For this review, take the finished solid that the model builds, in its own axes (mm). A direction names the side the tool comes from. Round coordinates to 2 decimals unless told otherwise and drop trailing zeros. Order: outer loops, then holes, each group sorted by start corner. A loop starts at its lowest first (then second) coordinate and runs counter-clockwise, first axis right, second up. Notation, with made-up numbers: M -36.75,42 L -19.75,42 A34 cw -19.75,72 Z; hole C -14,69.5 d3. An arc over 180 degrees is marked long. Put each result on its own line as item: value.
from build123d import *

# Parameters (mm, degrees)
BOSS_EXTRUDE1_DEPTH = 6.35


with BuildPart() as part:
    # Sketch1 → Boss-Extrude1 (new body)
    with BuildSketch(Plane(origin=(0, 0, 0), x_dir=(1, 0, 0), z_dir=(0, 1, 0))):
        with BuildLine():
            ThreePointArc((11.585828754, -34.373994235), (16.841756292, -62.617220967), (31.905828754, -87.078994235))
            Line((31.905828754, -87.078994235), (31.905828754, 39.921005765))
            Line((31.905828754, 39.921005765), (-120.494171246, 39.921005765))
            Line((-120.494171246, 39.921005765), (-120.494171246, -87.078994235))
            ThreePointArc((-120.494171246, -87.078994235), (-105.430098785, -62.617220967), (-100.174171246, -34.373994235))
            ThreePointArc((-100.174171246, -34.373994235), (-44.294171246, 21.506005765), (11.585828754, -34.373994235))
        make_face()
        with BuildLine():
            Line((31.905828754, 39.921005765), (31.905828754, -87.078994235))
            ThreePointArc((31.905828754, -87.078994235), (46.969901215, -62.617220967), (52.225828754, -34.373994235))
            ThreePointArc((52.225828754, -34.373994235), (108.105828754, 21.506005765), (163.985828754, -34.373994235))
            ThreePointArc((163.985828754, -34.373994235), (169.241756292, -62.617220967), (184.305828754, -87.078994235))
            Line((184.305828754, -87.078994235), (184.305828754, 39.921005765))
            Line((184.305828754, 39.921005765), (31.905828754, 39.921005765))
        make_face()
        with BuildLine():
            Line((336.705828754, 39.921005765), (184.305828754, 39.921005765))
            Line((184.305828754, 39.921005765), (184.305828754, -87.078994235))
            ThreePointArc((184.305828754, -87.078994235), (199.369901215, -62.617220967), (204.625828754, -34.373994235))
            ThreePointArc((204.625828754, -34.373994235), (260.505828754, 21.506005765), (316.385828754, -34.373994235))
            ThreePointArc((316.385828754, -34.373994235), (321.641756292, -62.617220967), (336.705828754, -87.078994235))
            Line((336.705828754, -87.078994235), (336.705828754, 39.921005765))
        make_face()
    extrude(amount=-BOSS_EXTRUDE1_DEPTH)


solid = part.part
(1) Add section B-B on y = -3.25. Give the boundary of the cut face in (x, z).
A:
outline: M -120.49,-39.92 L 336.71,-39.92 L 336.71,87.08 A78.51 ccw 316.39,34.37 A55.88 cw 204.63,34.37 A78.51 ccw 184.31,87.08 A78.51 ccw 163.99,34.37 A55.88 cw 52.23,34.37 A78.51 ccw 31.91,87.08 A78.51 ccw 11.59,34.37 A55.88 cw -100.17,34.37 A78.51 ccw -120.49,87.08 Z
(2) Add section C-C on z = -16. Give the boundary of the cut face in (x, y), then the cut area to 3 significant figures.
A:
outline: M -120.49,-6.35 L -68.48,-6.35 L -68.48,0 L -120.49,0 Z; M -20.11,-6.35 L 83.92,-6.35 L 83.92,0 L -20.11,0 Z; M 132.29,-6.35 L 236.32,-6.35 L 236.32,0 L 132.29,0 Z; M 284.69,-6.35 L 336.71,-6.35 L 336.71,0 L 284.69,0 Z
area: 1,980 mm2
(3) For faces 4 (the face through (107, -6.35, -28)), 5 (the face through (321.497, -3.131, 62.239)), list the 3-axis set-ups (+Z, -Z, +X, -X, +Y, -Y) from which the entire face can be reached by the end or side of a thin tool; tool diameter is ignored.
A:
face 4: +Z, -Z, +X, -X, -Y
face 5: +Z, +Y, -Y
(4) Draft analysis for pull direction X (two halves, no side actions). For faces 1 (the face through (-45.523, -3.131, -21.492)), 2 (the face through (107, 0, -28)), 3 (the face through (169.097, -3.131, 62.239)), state which applies: released by +X, released by -X, zero draft, split by the parting line, or undercut.
A:
face 1: undercut
face 2: zero draft
face 3: undercut
(5) To check wall thickness, follow L1, parallel to X at y = -3, z = 51; L2, parallel to X at y = -3, z = 66; L3, parallel to Z at x = 270, y = -2.75. State the ranges of each line that lie inside material, in increasing order.
A:
L1: x = -120.49 to -101.95, 13.37 to 50.45, 165.77 to 202.85, 318.17 to 336.71
L2: x = -120.49 to -106.83, 18.24 to 45.57, 170.64 to 197.97, 323.04 to 336.71
L3: z = -39.92 to -20.69
(6) Add section D-D on x = 87.5. Give the boundary of the cut face in (y, z).
A:
outline: M -6.35,-39.92 L 0,-39.92 L 0,-17.57 L -6.35,-17.57 Z
(7) Add section A-A on z = 50. Give the boundary of the cut face in (x, y), then the cut area to 3 significant figures.
A:
outline: M -120.49,-6.35 L -101.74,-6.35 L -101.74,0 L -120.49,0 Z; M 13.16,-6.35 L 50.66,-6.35 L 50.66,0 L 13.16,0 Z; M 165.56,-6.35 L 203.06,-6.35 L 203.06,0 L 165.56,0 Z; M 317.96,-6.35 L 336.71,-6.35 L 336.71,0 L 317.96,0 Z
area: 714 mm2
